Verification items for the finished model (mm, model axes). A direction names the side the tool comes from. Give positions to 0.01 mm unless a question says otherwise; leave off trailing zeros. Write each loop counter-clockwise with the first axis right and the second up, starting at its lowest first coordinate (ties: lowest second). Pieces come first, ordered by that corner, then holes. Notation, with made-up numbers: (70.25, 20.25) -> (90.25, 20.25) arc R6 ccw to (90.25, 28.25) -> close; hole circle Ø3 at (79.5, -8). An arc over 180 degrees is marked (long way). Write item = value, one per line.
from build123d import *

# Parameters (mm, degrees)
SKETCH_1_R      = 6
SKETCH_1_R_2    = 2.25
EXTRUDE_1_DEPTH = 10
SKETCH_2_R      = 12
SKETCH_2_R_2    = 6
EXTRUDE_2_DEPTH = 30
CHAMFER_1_SIZE  = 1


with BuildPart() as part:
    # 草图1 → 凸台-拉伸1 (new body)
    with BuildSketch(Plane(origin=(0, 0, 0), x_dir=(1, 0, 0), z_dir=(0, 1, 0))):
        with BuildLine():
            Line((-15, 13.228756555), (-15, -13.228756555))
            ThreePointArc((-15, -13.228756555), (0, -20), (15, -13.228756555))
            Line((15, -13.228756555), (15, 13.228756555))
            ThreePointArc((15, 13.228756555), (0, 20), (-15, 13.228756555))
        make_face()
        with Locations(Location((0, 0, 0), (0, 0, 270))):
            Circle(SKETCH_1_R, mode=Mode.SUBTRACT)
        with Locations(Location((0, 16, 0), (0, 0, 270))):
            Circle(SKETCH_1_R_2, mode=Mode.SUBTRACT)
        with Locations(Location((11.313708499, 11.313708499, 0), (0, 0, 270))):
            Circle(SKETCH_1_R_2, mode=Mode.SUBTRACT)
        with Locations(Location((-11.313708499, 11.313708499, 0), (0, 0, 90))):
            Circle(SKETCH_1_R_2, mode=Mode.SUBTRACT)
        with Locations(Location((-11.313708499, -11.313708499, 0), (0, 0, 270))):
            Circle(SKETCH_1_R_2, mode=Mode.SUBTRACT)
        with Locations(Location((0, -16, 0), (0, 0, 90))):
            Circle(SKETCH_1_R_2, mode=Mode.SUBTRACT)
        with Locations(Location((11.313708499, -11.313708499, 0), (0, 0, 90))):
            Circle(SKETCH_1_R_2, mode=Mode.SUBTRACT)
    extrude(amount=EXTRUDE_1_DEPTH)

    # 草图2 → 凸台-拉伸2 (add)
    with BuildSketch(Plane(origin=(0, 10, 0), x_dir=(1, 0, 0), z_dir=(0, 1, 0))):
        with Locations(Location((0, 0, 0), (0, 0, 90))):
            Circle(SKETCH_2_R)
        with Locations(Location((0, 0, 0), (0, 0, 270))):
            Circle(SKETCH_2_R_2, mode=Mode.SUBTRACT)
    extrude(amount=EXTRUDE_2_DEPTH)

    # 倒角1
    chamfer_1_edges = [part.edges().sort_by_distance(p)[0] for p in [
        (0, 40, 12),
    ]]
    chamfer(chamfer_1_edges, length=CHAMFER_1_SIZE)


solid = part.part
Item 1: Sectioned sample at C-C on y = 36. Record the cut outline in (x, z).
Response values:
outline = circle Ø24 at (0, 0); hole circle Ø12 at (0, 0)
Item 2: Sectioned sample at B-B on x = 0. Record the cut outline in (y, z).
Response values:
outline = (0, -20) -> (10, -20) -> (10, -18.25) -> (0, -18.25) -> close; (0, -13.75) -> (10, -13.75) -> (10, -12) -> (39, -12) -> (40, -11) -> (40, -6) -> (0, -6) -> close; (0, 6) -> (40, 6) -> (40, 11) -> (39, 12) -> (10, 12) -> (10, 13.75) -> (0, 13.75) -> close; (0, 18.25) -> (10, 18.25) -> (10, 20) -> (0, 20) -> close
Item 3: Go/stop test with flat-tipped pins: P1, Ø6, axis at x = 11.31, z = 11.31, coming from the +Y side; P2, Ø3.5, axis at x = -11.31, z = -11.31, coming from the -Y side; P3, Ø5, axis at x = 11, y = 28.5, coming from the +Z side; P4, Ø12, axis at x = -7, y = 35.5, coming from the -Z side. Record where each tip stops, or that it passes through.
Response values:
P1 = 10
P2 = through
P3 = 8.47
P4 = -11.96
Item 4: Sectioned sample at A-A on z = 16. Record the cut outline in (x, y), then the cut area to 3 significant figures.
Response values:
outline = (-12, 0) -> (-2.25, 0) -> (-2.25, 10) -> (-12, 10) -> close; (2.25, 0) -> (12, 0) -> (12, 10) -> (2.25, 10) -> close
area = 195 mm^2
Item 5: Set-up check for faces 1 (the cylindrical face through (-3.604, 24.297, -11.446)), 2 (the flat face through (6.5, 0, -0.3)): record each of +Z, -Z, +X, -X, +Y, -Y from which the full face is reachable in a straight line by a thin tool's end or side.
Response values:
face_1 = +Y
face_2 = +Z, -Z, +X, -X, -Y
Item 6: Mould release check, pull along Z, two halves, no side actions. Record for faces 3 (the flat face through (15, 5, 0)), 4 (the cylindrical face through (1.802, 19.72, 5.723)), 5 (the cylindrical face through (0, 5, 20)), 6 (the cylindrical face through (-13.211, 4.93, -12.523)): +Z half, -Z half, draft (parallel to the pull), parting line (faces both ways), or undercut.
Response values:
face_3 = draft
face_4 = undercut
face_5 = +Z half
face_6 = undercut
Item 7: Material ranges on line 1 (X direction, y = 25.5, z = 0); line 2 (X direction, y = 4, z = 16); line 3 (Y direction, x = 12.25, z = -5), recorded low to high.
Response values:
line_1 = -12 to -6, 6 to 12
line_2 = -12 to -2.25, 2.25 to 12
line_3 = 0 to 10
Item 8: Sectioned sample at D-D on z = 0. Record the cut outline in (x, y).
Response values:
outline = (-15, 0) -> (-6, 0) -> (-6, 40) -> (-11, 40) -> (-12, 39) -> (-12, 10) -> (-15, 10) -> close; (6, 0) -> (15, 0) -> (15, 10) -> (12, 10) -> (12, 39) -> (11, 40) -> (6, 40) -> close
